The drawing under review shows one solid part. Ordinate dimensions are in mm from its lowest x, y, z. A direction names the side the tool comes from. Round coordinates to 2 decimals unless told otherwise and drop trailing zeros. Loops run counter-clockwise (first coordinate to the right, second up) from the corner with the lowest first, then second, coordinate; pieces in that order, holes last. Notation, with made-up numbers: (33, 38) - (63, 38) arc R15 cw to (63, 65) - close; hole circle Ø11 at (65, 67). An arc over 180 degrees is marked (long way). Answer as CSV lines item,"result".
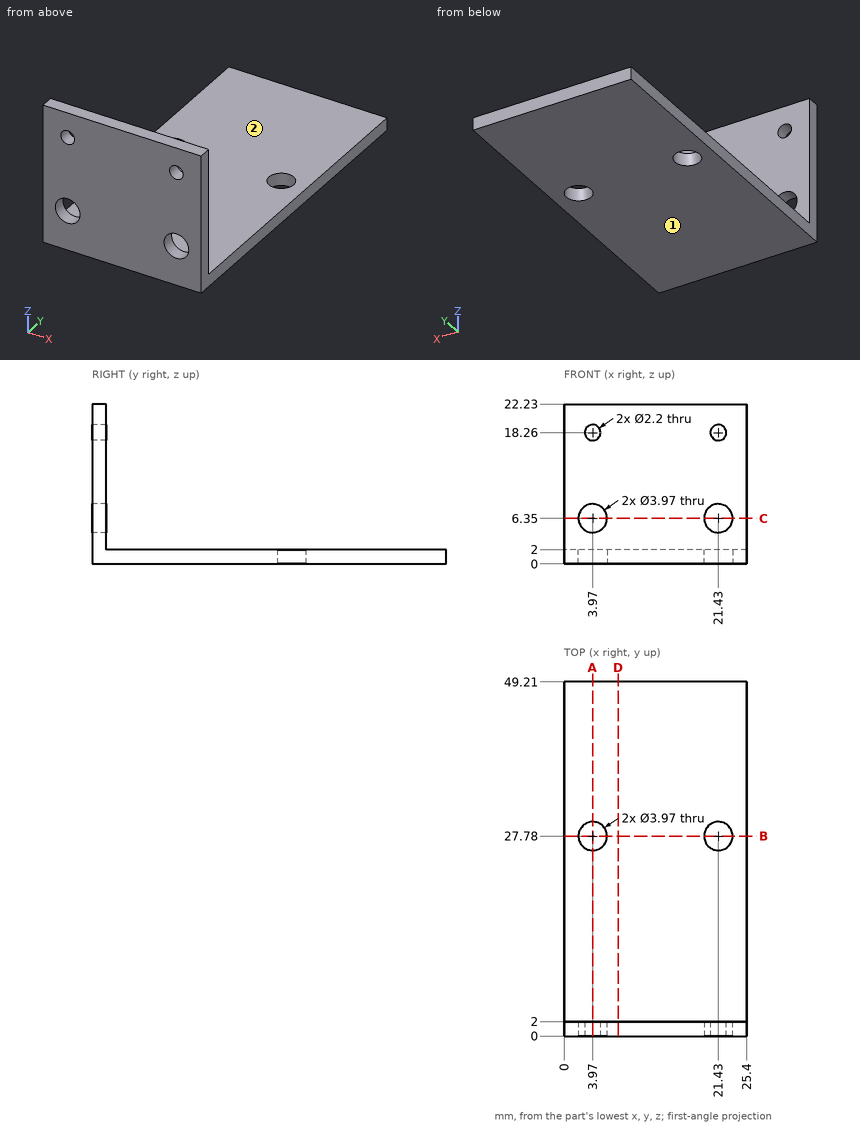
1. Clearance check with flat-ended pins moving along their axes: pin 1 (2.5 mm diameter, centred on x = 21.43, z = 6.35, fed in from -Y); pin 2 (4.5 mm diameter, centred on x = 3.97, y = 27.78, fed in from +Z); pin 3 (8 mm diameter, centred on x = 11.5, z = 18.5, fed in from +Y). State where each tip first meets the part, or that it passes through.
Numbers:
pin 1,"passes through"
pin 2,"stops at z = 2"
pin 3,"stops at y = 2"
2. Tool access review of the marked faces 1 and 2: name each direction out of +Z, -Z, +X, -X, +Y, -Y from which nothing blocks a thin tool from reaching the whole face with its end or side.
Numbers:
face 1,"-Z, +X, -X, +Y, -Y"
face 2,"+Z, +X, -X, +Y"
3. Take a section at A-A (x = 3.97). State the section outline as (y, z) points (3 decimals), plus the area to 3 significant figures.
Numbers:
outline,"(0, 0) - (25.795, 0) - (25.795, 2) - (2, 2) - (2, 4.365) - (0, 4.365) - close; (0, 8.335) - (2, 8.335) - (2, 17.16) - (0, 17.16) - close; (0, 19.36) - (2, 19.36) - (2, 22.23) - (0, 22.23) - close; (29.765, 0) - (49.21, 0) - (49.21, 2) - (29.765, 2) - close"
area,"119 mm²"
4. Take a section at B-B (y = 27.78). State the section outline as (x, z) points (3 decimals), plus the area to 3 significant figures.
Numbers:
outline,"(0, 0) - (1.985, 0) - (1.985, 2) - (0, 2) - close; (5.955, 0) - (19.445, 0) - (19.445, 2) - (5.955, 2) - close; (23.415, 0) - (25.4, 0) - (25.4, 2) - (23.415, 2) - close"
area,"34.9 mm²"
5. Wall thickness on probe 1 along Z at (x, y) = (21.43, 1) (3 decimals); probe 2 along X at (y, z) = (1.2, 18.26); probe 3 along Z at (x, y) = (13.25, 35): over which ranges is each line inside the solid? List them lowest first.
Numbers:
probe 1,"z = 0 to 4.365, 8.335 to 17.16, 19.36 to 22.23"
probe 2,"x = 0 to 2.87, 5.07 to 20.33, 22.53 to 25.4"
probe 3,"z = 0 to 2"
6. Take a section at D-D (x = 7.5). State the section outline as (y, z) points, plus the area to 3 significant figures.
Numbers:
outline,"(0, 0) - (49.21, 0) - (49.21, 2) - (2, 2) - (2, 22.23) - (0, 22.23) - close"
area,"139 mm²"
